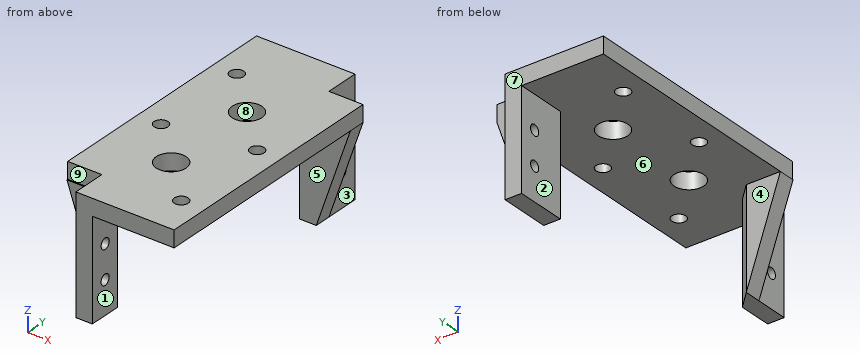
from build123d import *

# Parameters (mm, degrees)
SKETCH1_W           = 80
SKETCH1_H           = 85
BOSS_EXTRUDE1_DEPTH = 5
CUT_EXTRUDE1_REACH  = 60.577
SKETCH2_R           = 4.5
SKETCH2_R_2         = 2.1
CUT_EXTRUDE2_REACH  = 60.577
SKETCH3_W           = 10.3
SKETCH3_H           = 10.3
SKETCH3_W_2         = 10
SKETCH3_H_2         = 10
SKETCH4_W           = 40
SKETCH4_H           = 85
CUT_EXTRUDE4_DEPTH  = 10
SKETCH5_W           = 5
SKETCH5_H           = 10.3
BOSS_EXTRUDE2_DEPTH = 30
BOSS_EXTRUDE3_DEPTH = 5
CUT_EXTRUDE5_REACH  = 67.622
SKETCH7_W           = 10.3
SKETCH7_H           = 10.3
SKETCH8_W           = 5
SKETCH8_H           = 15
BOSS_EXTRUDE4_DEPTH = 30
BOSS_EXTRUDE5_DEPTH = 5
CHAMFER1_SIZE       = 5
CUT_EXTRUDE6_REACH  = 61.903
SKETCH10_R          = 1.6
CUT_EXTRUDE7_REACH  = 61.903
SKETCH12_R          = 1.6


with BuildPart() as part:
    # Sketch1 → Boss-Extrude1 (new body)
    with BuildSketch(Plane.XY):
        Rectangle(SKETCH1_W, SKETCH1_H)
    extrude(amount=BOSS_EXTRUDE1_DEPTH)

    # Sketch2 → Cut-Extrude1 (cut, up to next)
    with BuildSketch(Plane(origin=(0, 0, 0), x_dir=(-1, 0, 0), z_dir=(0, 0, -1)), mode=Mode.PRIVATE) as cut_extrude1_sk1:
        with Locations((-20, 12.5)):
            Circle(SKETCH2_R)
    cut_extrude1_tool1 = extrude(cut_extrude1_sk1.sketch, amount=-CUT_EXTRUDE1_REACH, mode=Mode.PRIVATE) & part.part
    # Sketch2 → Cut-Extrude1 (cut, up to next)
    with BuildSketch(Plane(origin=(0, 0, 0), x_dir=(-1, 0, 0), z_dir=(0, 0, -1)), mode=Mode.PRIVATE) as cut_extrude1_sk2:
        with Locations((-7.095301243, 25.404698757)):
            Circle(SKETCH2_R_2)
    cut_extrude1_tool2 = extrude(cut_extrude1_sk2.sketch, amount=-CUT_EXTRUDE1_REACH, mode=Mode.PRIVATE) & part.part
    # Sketch2 → Cut-Extrude1 (cut, up to next)
    with BuildSketch(Plane(origin=(0, 0, 0), x_dir=(-1, 0, 0), z_dir=(0, 0, -1)), mode=Mode.PRIVATE) as cut_extrude1_sk3:
        with Locations((-32.904698757, -0.404698757)):
            Circle(SKETCH2_R_2)
    cut_extrude1_tool3 = extrude(cut_extrude1_sk3.sketch, amount=-CUT_EXTRUDE1_REACH, mode=Mode.PRIVATE) & part.part
    # Sketch2 → Cut-Extrude1 (cut, up to next)
    with BuildSketch(Plane(origin=(0, 0, 0), x_dir=(-1, 0, 0), z_dir=(0, 0, -1)), mode=Mode.PRIVATE) as cut_extrude1_sk4:
        with Locations((-20, -17.5)):
            Circle(SKETCH2_R)
    cut_extrude1_tool4 = extrude(cut_extrude1_sk4.sketch, amount=-CUT_EXTRUDE1_REACH, mode=Mode.PRIVATE) & part.part
    # Sketch2 → Cut-Extrude1 (cut, up to next)
    with BuildSketch(Plane(origin=(0, 0, 0), x_dir=(-1, 0, 0), z_dir=(0, 0, -1)), mode=Mode.PRIVATE) as cut_extrude1_sk5:
        with Locations((-7.095301243, -4.595301243)):
            Circle(SKETCH2_R_2)
    cut_extrude1_tool5 = extrude(cut_extrude1_sk5.sketch, amount=-CUT_EXTRUDE1_REACH, mode=Mode.PRIVATE) & part.part
    # Sketch2 → Cut-Extrude1 (cut, up to next)
    with BuildSketch(Plane(origin=(0, 0, 0), x_dir=(-1, 0, 0), z_dir=(0, 0, -1)), mode=Mode.PRIVATE) as cut_extrude1_sk6:
        with Locations((-32.904698757, -30.404698757)):
            Circle(SKETCH2_R_2)
    cut_extrude1_tool6 = extrude(cut_extrude1_sk6.sketch, amount=-CUT_EXTRUDE1_REACH, mode=Mode.PRIVATE) & part.part
    add(cut_extrude1_tool1.solids().sort_by_distance((20, 12.5, 0))[0], mode=Mode.SUBTRACT)
    add(cut_extrude1_tool2.solids().sort_by_distance((7.095301, 25.404699, 0))[0], mode=Mode.SUBTRACT)
    add(cut_extrude1_tool3.solids().sort_by_distance((32.904699, -0.404699, 0))[0], mode=Mode.SUBTRACT)
    add(cut_extrude1_tool4.solids().sort_by_distance((20, -17.5, 0))[0], mode=Mode.SUBTRACT)
    add(cut_extrude1_tool5.solids().sort_by_distance((7.095301, -4.595301, 0))[0], mode=Mode.SUBTRACT)
    add(cut_extrude1_tool6.solids().sort_by_distance((32.904699, -30.404699, 0))[0], mode=Mode.SUBTRACT)

    # Sketch3 → Cut-Extrude2 (cut, up to next)
    with BuildSketch(Plane(origin=(0, 0, 0), x_dir=(-1, 0, 0), z_dir=(0, 0, -1)), mode=Mode.PRIVATE) as cut_extrude2_sk1:
        with Locations((-34.85, 37.35)):
            Rectangle(SKETCH3_W, SKETCH3_H)
    cut_extrude2_tool1 = extrude(cut_extrude2_sk1.sketch, amount=-CUT_EXTRUDE2_REACH, mode=Mode.PRIVATE) & part.part
    # Sketch3 → Cut-Extrude2 (cut, up to next)
    with BuildSketch(Plane(origin=(0, 0, 0), x_dir=(-1, 0, 0), z_dir=(0, 0, -1)), mode=Mode.PRIVATE) as cut_extrude2_sk2:
        with Locations((35, 37.5)):
            Rectangle(SKETCH3_W_2, SKETCH3_H_2)
    cut_extrude2_tool2 = extrude(cut_extrude2_sk2.sketch, amount=-CUT_EXTRUDE2_REACH, mode=Mode.PRIVATE) & part.part
    add(cut_extrude2_tool1.solids().sort_by_distance((34.85, 37.35, 0))[0], mode=Mode.SUBTRACT)
    add(cut_extrude2_tool2.solids().sort_by_distance((-35, 37.5, 0))[0], mode=Mode.SUBTRACT)

    # Sketch4 → Cut-Extrude4 (cut)
    with BuildSketch(Plane(origin=(0, 0, 0), x_dir=(-1, 0, 0), z_dir=(0, 0, -1))):
        with Locations((20, 0)):
            Rectangle(SKETCH4_W, SKETCH4_H)
    extrude(amount=-CUT_EXTRUDE4_DEPTH, mode=Mode.SUBTRACT)

    # Sketch5 → Boss-Extrude2 (add)
    with BuildSketch(Plane(origin=(0, 0, 0), x_dir=(-1, 0, 0), z_dir=(0, 0, -1))):
        with Locations((-27.2, 37.35)):
            Rectangle(SKETCH5_W, SKETCH5_H)
    extrude(amount=BOSS_EXTRUDE2_DEPTH)

    # Sketch6 → Boss-Extrude3 (add)
    with BuildSketch(Plane.XZ.offset(-32.2)):
        Polygon((40, 0), (29.7, -30), (24.7, -30), (24.7, 5), (40, 5), align=None)
    extrude(amount=BOSS_EXTRUDE3_DEPTH)

    # Sketch7 → Cut-Extrude5 (cut, up to next)
    with BuildSketch(Plane(origin=(0, 0, 0), x_dir=(-1, 0, 0), z_dir=(0, 0, -1)), mode=Mode.PRIVATE) as cut_extrude5_sk1:
        with Locations((-5.15, -37.35)):
            Rectangle(SKETCH7_W, SKETCH7_H)
    cut_extrude5_tool1 = extrude(cut_extrude5_sk1.sketch, amount=-CUT_EXTRUDE5_REACH, mode=Mode.PRIVATE) & part.part
    add(cut_extrude5_tool1.solids().sort_by_distance((5.15, -37.35, 0))[0], mode=Mode.SUBTRACT)

    # Sketch8 → Boss-Extrude4 (add)
    with BuildSketch(Plane(origin=(0, 0, 0), x_dir=(-1, 0, 0), z_dir=(0, 0, -1))):
        with Locations((-12.8, -35)):
            Rectangle(SKETCH8_W, SKETCH8_H)
    extrude(amount=BOSS_EXTRUDE4_DEPTH)

    # Sketch9 → Boss-Extrude5 (add)
    with BuildSketch(Plane(origin=(0, -27.5, 0), x_dir=(1, 0, 0), z_dir=(0, 1, 0))):
        Polygon((10.3, 30), (0, 0), (10.3, 0), align=None)
    extrude(amount=-BOSS_EXTRUDE5_DEPTH)

    # Chamfer1
    chamfer1_edges = [part.edges().sort_by_distance(p)[0] for p in [
        (15.3, -27.5, -15),
    ]]
    chamfer(chamfer1_edges, length=CHAMFER1_SIZE)

    # Sketch10 → Cut-Extrude6 (cut, up to next)
    with BuildSketch(Plane.ZY.offset(-10.3), mode=Mode.PRIVATE) as cut_extrude6_sk1:
        with Locations((-20, -37.457142857)):
            Circle(SKETCH10_R)
    cut_extrude6_tool1 = extrude(cut_extrude6_sk1.sketch, amount=-CUT_EXTRUDE6_REACH, mode=Mode.PRIVATE) & part.part
    # Sketch10 → Cut-Extrude6 (cut, up to next)
    with BuildSketch(Plane.ZY.offset(-10.3), mode=Mode.PRIVATE) as cut_extrude6_sk2:
        with Locations((-10, -37.414285714)):
            Circle(SKETCH10_R)
    cut_extrude6_tool2 = extrude(cut_extrude6_sk2.sketch, amount=-CUT_EXTRUDE6_REACH, mode=Mode.PRIVATE) & part.part
    add(cut_extrude6_tool1.solids().sort_by_distance((10.3, -37.457143, -20))[0], mode=Mode.SUBTRACT)
    add(cut_extrude6_tool2.solids().sort_by_distance((10.3, -37.414286, -10))[0], mode=Mode.SUBTRACT)

    # Sketch12 → Cut-Extrude7 (cut, up to next)
    with BuildSketch(Plane(origin=(29.7, 0, 0), x_dir=(0, 0, -1), z_dir=(1, 0, 0)), mode=Mode.PRIVATE) as cut_extrude7_sk1:
        with Locations(Location((20, 37.35, 0), (0, 0, 90))):
            Circle(SKETCH12_R)
    cut_extrude7_tool1 = extrude(cut_extrude7_sk1.sketch, amount=-CUT_EXTRUDE7_REACH, mode=Mode.PRIVATE) & part.part
    # Sketch12 → Cut-Extrude7 (cut, up to next)
    with BuildSketch(Plane(origin=(29.7, 0, 0), x_dir=(0, 0, -1), z_dir=(1, 0, 0)), mode=Mode.PRIVATE) as cut_extrude7_sk2:
        with Locations(Location((10, 37.35, 0), (0, 0, 90))):
            Circle(SKETCH12_R)
    cut_extrude7_tool2 = extrude(cut_extrude7_sk2.sketch, amount=-CUT_EXTRUDE7_REACH, mode=Mode.PRIVATE) & part.part
    add(cut_extrude7_tool1.solids().sort_by_distance((29.7, 37.35, -20))[0], mode=Mode.SUBTRACT)
    add(cut_extrude7_tool2.solids().sort_by_distance((29.7, 37.35, -10))[0], mode=Mode.SUBTRACT)


solid = part.part
Part model, mm, in its own coordinate system. Face numbers are marked on the shaded views. A direction names the side the tool comes from. Give positions to 0.01 mm unless a question says otherwise; leave off trailing zeros. Write each loop counter-clockwise with the first axis right and the second up, starting at its lowest first coordinate (ties: lowest second). Pieces come first, ordered by that corner, then holes.
1) Cut at A-A on z = -6. Write the cut outline in (x, y).
Resolved:
outline: (2.06, -32.5) - (10.3, -32.5) - (10.3, -42.5) - (15.3, -42.5) - (15.3, -32.5) - (10.3, -27.5) - (2.06, -27.5) - close; (24.7, 27.2) - (37.94, 27.2) - (37.94, 32.2) - (29.7, 32.2) - (29.7, 42.5) - (24.7, 42.5) - close
2) Cut at C-C on y = 37.35. Write the cut outline in (x, z), then the cut area to 4 significant figures.
Resolved:
outline: (0, 0) - (24.7, 0) - (24.7, -8.4) - (29.7, -8.4) - (29.7, 5) - (0, 5) - close; (24.7, -30) - (29.7, -30) - (29.7, -21.6) - (24.7, -21.6) - close; (24.7, -18.4) - (29.7, -18.4) - (29.7, -11.6) - (24.7, -11.6) - close
area: 266.5 mm2
3) Pin check, flat tips, straight feed: pin 1 (8 mm diameter, centred on x = 5.5, z = -11, fed in from +Y); pin 2 (3 mm diameter, centred on y = 37.5, z = -18, fed in from +X); pin 3 (10 mm diameter, centred on y = -18, z = -26, fed in from +X); pin 4 (3.5 mm diameter, centred on y = -37.41, z = -10, fed in from -X). Stop position of each tip, or through.
Resolved:
pin 1: stops at y = -27.5
pin 2: stops at x = 29.7
pin 3: passes through
pin 4: stops at x = 10.3
4) Which spindle directions (+Z, -Z, +X, -X, +Y, -Y) get a long thin tool onto all of the face, cutting with end or side? Do the marked faces 1, 2, 3, 4 and 5. Say none if no direction does.
Resolved:
face 1: -Z, +X, +Y, -Y
face 2: -Z, -X, +Y, -Y
face 3: +Z, -Z, +X, +Y
face 4: -Z, +X, -X, +Y
face 5: -Z, +X, -X, -Y
5) Cut at D-D on y = -15.5. Write the cut outline in (x, z), then the cut area to 3 significant figures.
Resolved:
outline: (0, 0) - (15.97, 0) - (15.97, 5) - (0, 5) - close; (24.03, 0) - (40, 0) - (40, 5) - (24.03, 5) - close
area: 160 mm2
6) Two-plate mould, pull along Y, no slides. Class the marked faces 6, 7, 8 and 9: released by +Y, released by -Y, zero draft, split by the parting line, or undercut.
Resolved:
face 6: zero draft
face 7: released by +Y
face 8: undercut
face 9: released by -Y
7) Probe L1, parallel to Y at x = 20, z = 1.6; L2, parallel to Y at x = 12.8, z = -20; L3, parallel to X at y = 33.5, z = -27. List the from-to ranges inside material, lowest first.
Resolved:
L1: y = -42.5 to -22, -13 to 8, 17 to 42.5
L2: y = -42.5 to -39.06, -35.86 to -30
L3: x = 24.7 to 29.7
8) Cut at B-B on x = 28.5. Write the cut outline in (y, z), then the cut area to 3 significant figures.
Resolved:
outline: (-42.5, 0) - (27.2, 0) - (27.2, -30) - (42.5, -30) - (42.5, 5) - (-42.5, 5) - close; hole circle Ø3.2 at (37.35, -20); hole circle Ø3.2 at (37.35, -10)
area: 868 mm2
